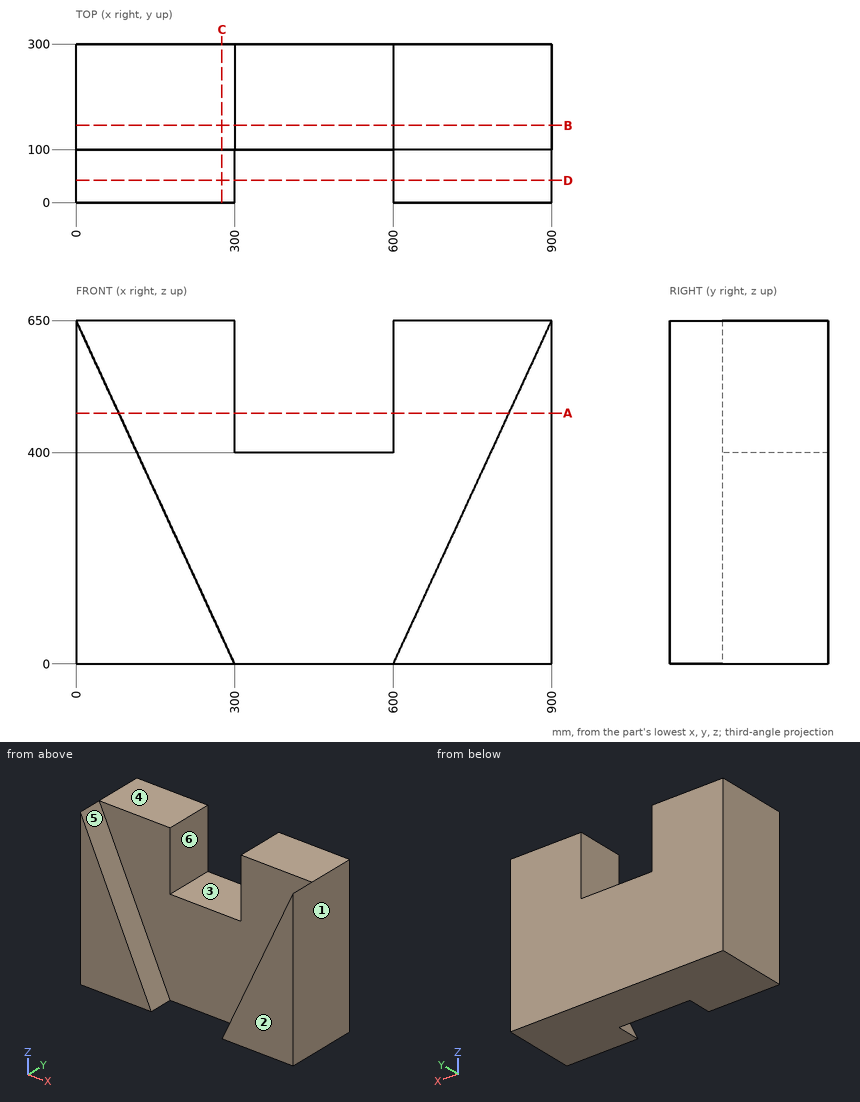
For this review, use the dimensioned drawing (mm, ordinates from the lowest corner) and the shaded views. A direction names the side the tool comes from. Round coordinates to 2 decimals unless told otherwise and drop trailing zeros. Write each loop counter-clockwise with the first axis right and the second up, starting at its lowest first coordinate (ties: lowest second). Pieces come first, ordered by that corner, then holes. Notation, with made-up numbers: (61, 69.25) - (119, 69.25) arc R20 cw to (119, 95.25) - close; hole circle Ø4 at (-6.75, 53.5). An arc over 180 degrees is marked (long way). Answer as a JSON object with one key per item and string values.
1. We need section B-B on y = 146. Give the boundary of the cut face in (x, z).
Response values:
{"outline": "(0, 0) - (900, 0) - (900, 650) - (600, 650) - (600, 400) - (300, 400) - (300, 650) - (0, 650) - close"}
2. We need section D-D on y = 42. Give the boundary of the cut face in (x, z), then the cut area to 3 significant figures.
Response values:
{"outline": "(0, 0) - (300, 0) - (0, 650) - close; (600, 0) - (900, 0) - (900, 650) - close", "area": "195,000 mm2"}
3. We need section A-A on z = 474.5. Give the boundary of the cut face in (x, y).
Response values:
{"outline": "(0, 0) - (81, 0) - (81, 100) - (300, 100) - (300, 300) - (0, 300) - close; (600, 100) - (819, 100) - (819, 0) - (900, 0) - (900, 300) - (600, 300) - close"}
4. For pin 1 Ø4 at (x, y) = (289, 206.5) entering from -Z; pin 2 Ø12 at (x, y) = (695, 71.5) entering from +Z; pin 3 Ø2 at (x, y) = (476.5, 130.5) entering from +Z, all flat-tipped, find the tip position at first contact; note any pin that passes through.
Response values:
{"pin 1": "stops at z = 0", "pin 2": "stops at z = 218.83", "pin 3": "stops at z = 400"}
5. To check wall thickness, follow line 1 along X through (y, z) = (256.5, 563); line 2 along Y through (x, z) = (426, 210.5); line 3 along X through (y, z) = (13, 369.5). State the ranges of each line that lie inside material, in increasing order.
Response values:
{"line 1": "x = 0 to 300, 600 to 900", "line 2": "y = 100 to 300", "line 3": "x = 0 to 129.46, 770.54 to 900"}
6. Draft analysis for pull direction X (two halves, no side actions). For the marked faces 1, 2 and 3, state which applies: +X half, -X half, draft (parallel to the pull), parting line (faces both ways), or undercut.
Response values:
{"face 1": "+X half", "face 2": "draft", "face 3": "undercut"}
7. We need section C-C on x = 276. Give the boundary of the cut face in (y, z).
Response values:
{"outline": "(0, 0) - (300, 0) - (300, 650) - (100, 650) - (100, 52) - (0, 52) - close"}
8. Tool access review of the marked faces 4, 5 and 6: name each direction out of +Z, -Z, +X, -X, +Y, -Y from which nothing blocks a thin tool from reaching the whole face with its end or side.
Response values:
{"face 4": "+Z, +X, -X, +Y, -Y", "face 5": "+Z, -Y", "face 6": "+Z, +Y, -Y"}
